Build history of the part. All positions in model axes, mm. Round coordinates to 2 decimals unless told otherwise and drop trailing zeros. Write each loop counter-clockwise with the first axis right and the second up, starting at its lowest first coordinate (ties: lowest second). Pieces come first, ordered by that corner, then holes. Notation, with made-up numbers: M 53,-8.5 L 63,-8.5 A31 cw 63,25.5 Z; hole C 46,53 d4. An arc over 180 degrees is marked long. Use a Markdown table: item, result.
from build123d import *

# Parameters (mm, degrees)
SKETCH_2_R      = 26
EXTRUDE_1_DEPTH = 15
FILLET_1_R      = 5


with BuildPart() as part:
    # 草图1 → 旋转1 (revolve)
    with BuildSketch(Plane.XY):
        with BuildLine():
            Line((0, 0), (26, 0))
            Line((26, 0), (26, 1))
            ThreePointArc((26, 1), (25, 3), (26, 5))
            Line((26, 5), (26, 6))
            Line((26, 6), (0, 6))
            Line((0, 6), (0, 0))
        make_face()
    revolve(axis=Axis((0, 0, 0), (0, -1, 0)))

    # 草图2 → 凸台-拉伸1 (add)
    with BuildSketch(Plane(origin=(0, 6, 0), x_dir=(1, 0, 0), z_dir=(0, 1, 0))):
        Circle(SKETCH_2_R)
    extrude(amount=EXTRUDE_1_DEPTH)

    # 圆角1
    fillet_1_edges = [part.edges().sort_by_distance(p)[0] for p in [
        (-26, 21, 0),
    ]]
    fillet(fillet_1_edges, radius=FILLET_1_R)


solid = part.part
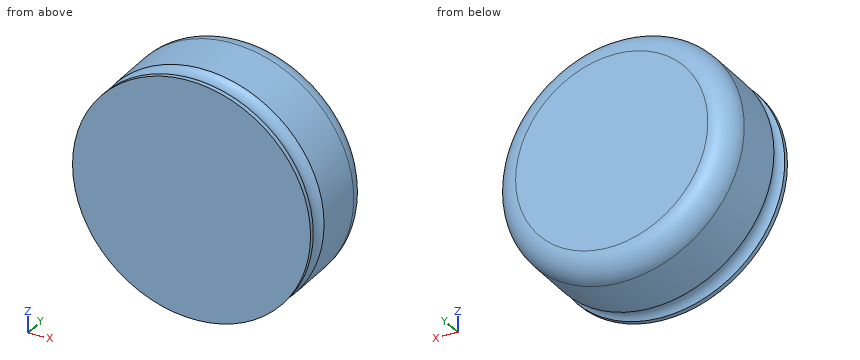
Q1. Cut at A-A on y = 15. Give the cut face in (x, z).
Response values:
| item | result |
|---|---|
| outline | C 0,0 d52 |
Q2. Cut at B-B on y = 18.5. Give the cut face in (x, z), and give its area (3 significant figures).
Response values:
| item | result |
|---|---|
| outline | C 0,0 d50.66 |
| area | 2,020 mm2 |
Q3. Drill centre lines: L1, parallel to X at y = 5.5, z = -0.5; L2, parallel to Z at x = 23.5, y = 9.5; L3, parallel to X at y = 16, z = 10. Where is each one in solid material? Low to high.
Response values:
| item | result |
|---|---|
| L1 | x = -26 to 26 |
| L2 | z = -11.12 to 11.12 |
| L3 | x = -24 to 24 |
Q4. Drop flat-ended pins along their axis: P1, Ø12, axis at y = 3.5, z = 10, coming from the +X side; P2, Ø8, axis at y = 14, z = -0.5, coming from the -X side; P3, Ø1, axis at x = 6, y = 13.5, coming from the -Z side; P4, Ø12, axis at x = 0.5, y = 13.5, coming from the -Z side. Give the stop position or say it passes through.
Response values:
| item | result |
|---|---|
| P1 | stops at x = 25.66 |
| P2 | stops at x = -26 |
| P3 | stops at z = -25.41 |
| P4 | stops at z = -26 |
